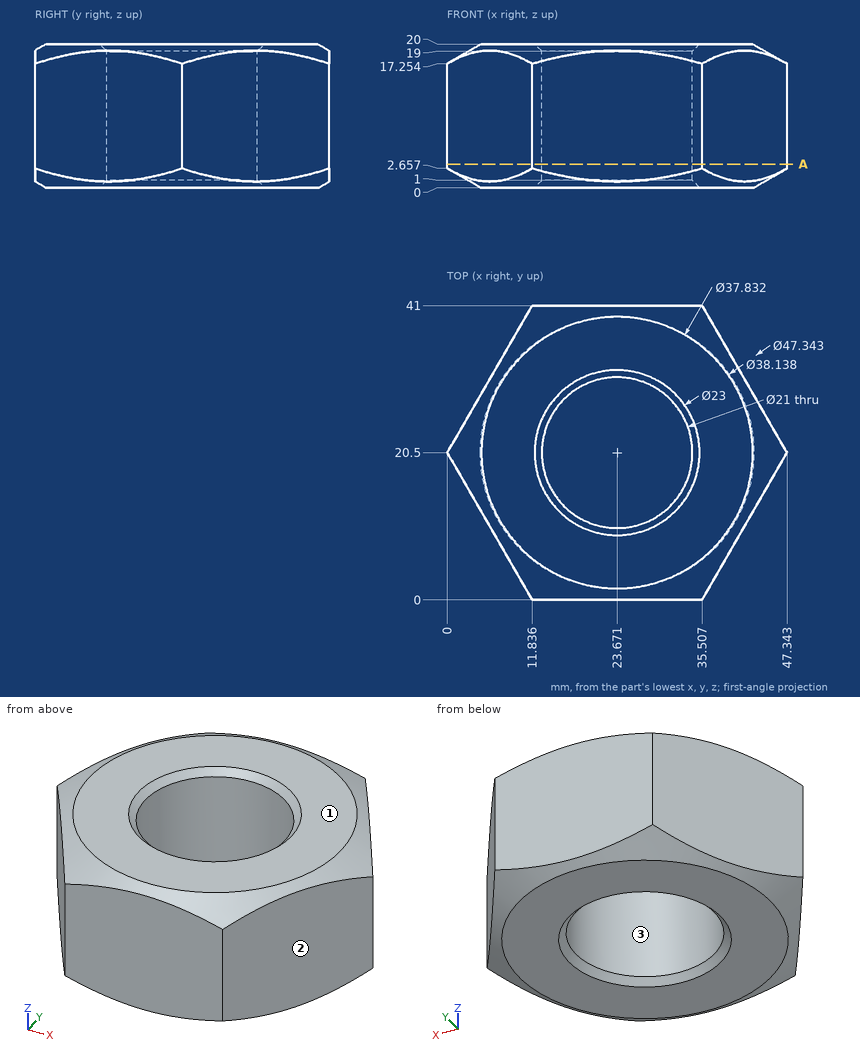
Answer from the drawing. Dimensions are ordinates in mm from the lowest x, y and z of the part. Give positions to 0.01 mm unless a question says otherwise; leave off trailing zeros. Loops run counter-clockwise (first coordinate to the right, second up) from the corner with the lowest first, then second, coordinate; pieces in that order, holes last. Notation, with made-up numbers: M 28.25,57.5 L 75.25,57.5 A23 ccw 75.25,95.5 Z; hole C -18,45.5 d1. An arc over 180 degrees is marked long. One line per item, written item: value.
Q1. Flat-ended cylindrical pins translate along their axes: P1, Ø3, axis at y = 10, z = 15, coming from the +X side; P2, Ø4, axis at x = 18, z = 7, coming from the -Y side. Find the tip coordinate at first contact, or state that the pin passes through.
Working result:
P1: stops at x = 42.15
P2: stops at y = 0
Q2. Find the intervals of material crossed by line 1 (Y direction, x = 23.5, z = 15.5); line 2 (Y direction, x = 31, z = 5.5); line 3 (X direction, y = 22, z = 11) (1 decimal), in increasing order. Write a range as from..to.
Working result:
line 1: y = 0..10, 31..41
line 2: y = 0..12.98, 28.02..41
line 3: x = 0.9..13.3, 34.1..46.5
Q3. Determine the mould class of the marked faces 1, 2 and 3 for opening direction Y: +Y half, -Y half, draft (parallel to the pull), parting line (faces both ways), or undercut.
Working result:
face 1: draft
face 2: -Y half
face 3: undercut
Q4. A cutting plane is placed at A-A on z = 3.25. Determine the outline of the cut face in (x, y) (1 decimal), then the cut area to 3 significant figures.
Working result:
outline: M 0,20.5 L 11.8,0 L 35.5,0 L 47.3,20.5 L 35.5,41 L 11.8,41 Z; hole C 23.7,20.5 d21
area: 1,110 mm^2
